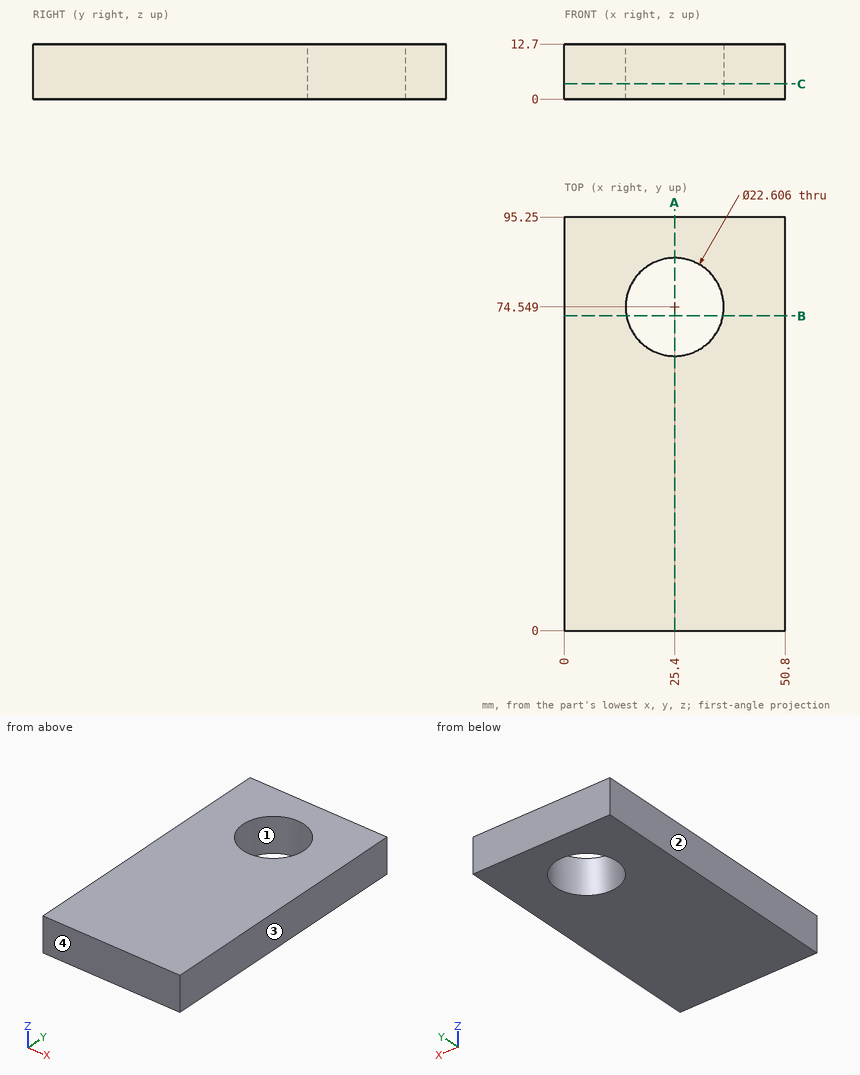
Drawing for the job (mm, zero at the part's lowest x, y, z). Give positions to 0.01 mm unless a question says otherwise; leave off trailing zeros. Loops run counter-clockwise (first coordinate to the right, second up) from the corner with the lowest first, then second, coordinate; pieces in that order, holes last.
Item 1: Drop a flat-ended pin along its axis: P1, Ø20.5, axis at x = 25.4, y = 74.549, coming from the -Z side. Give the stop position or say it passes through.
Check values:
P1: passes through
Item 2: Mould opens along X. For the marked faces 1, 2, 3 and 4 say: +X half, -X half, draft (parallel to the pull), parting line (faces both ways), or undercut.
Check values:
face 1: undercut
face 2: -X half
face 3: +X half
face 4: draft
Item 3: Slice it at C-C (z = 3.5). Write the cut outline in (x, y), plus the area to 3 significant figures.
Check values:
outline: (0, 0) - (50.8, 0) - (50.8, 95.25) - (0, 95.25) - close; hole circle Ø22.61 at (25.4, 74.55)
area: 4,440 mm2
Item 4: Slice it at B-B (y = 72.5). Write the cut outline in (x, z).
Check values:
outline: (0, 0) - (14.28, 0) - (14.28, 12.7) - (0, 12.7) - close; (36.52, 0) - (50.8, 0) - (50.8, 12.7) - (36.52, 12.7) - close
Item 5: Slice it at A-A (x = 25.4). Write the cut outline in (y, z), plus the area to 3 significant figures.
Check values:
outline: (0, 0) - (63.25, 0) - (63.25, 12.7) - (0, 12.7) - close; (85.85, 0) - (95.25, 0) - (95.25, 12.7) - (85.85, 12.7) - close
area: 923 mm2
Item 6: Drill centre lines: line 1 along Y through (x, z) = (25.4, 5.5); line 2 along X through (y, z) = (66.5, 7); line 3 along X through (y, z) = (69.5, 0.5). Where is each one in solid material? Low to high.
Check values:
line 1: y = 0 to 63.25, 85.85 to 95.25
line 2: x = 0 to 17.46, 33.34 to 50.8
line 3: x = 0 to 15.29, 35.51 to 50.8
